```python
from build123d import *

# Parameters (mm, degrees)
SKETCH1_R           = 10.1
BOSS_EXTRUDE1_DEPTH = 13
SKETCH2_R           = 14
BOSS_EXTRUDE2_DEPTH = 3
SKETCH3_R           = 2
CUT_EXTRUDE1_DEPTH  = 17
CIRPATTERN1_COUNT   = 4


with BuildPart() as part:
    # Sketch1 → Boss-Extrude1 (new body)
    with BuildSketch(Plane(origin=(0, 0, 0), x_dir=(1, 0, 0), z_dir=(0, 1, 0))):
        Circle(SKETCH1_R)
    extrude(amount=BOSS_EXTRUDE1_DEPTH)

    # Sketch2 → Boss-Extrude2 (add)
    with BuildSketch(Plane(origin=(0, 13, 0), x_dir=(1, 0, 0), z_dir=(0, 1, 0))):
        Circle(SKETCH2_R)
    extrude(amount=BOSS_EXTRUDE2_DEPTH)

    # Sketch3 → Cut-Extrude1 (cut, through all)
    with BuildSketch(Plane.XZ):
        with Locations((0, 6)):
            Circle(SKETCH3_R)
    cut_extrude1 = extrude(amount=-CUT_EXTRUDE1_DEPTH, mode=Mode.SUBTRACT)

    # CirPattern1: Cut-Extrude1 ×4 about axis
    cirpattern1_axis = Axis((0, 0, 0), (0, 1, 0))
    for i in range(1, CIRPATTERN1_COUNT):
        add(cut_extrude1.rotate(cirpattern1_axis, i * 360 / CIRPATTERN1_COUNT), mode=Mode.SUBTRACT)


solid = part.part
```
CAD build for the part. Positions are in the model's coordinates, mm. A direction names the side the tool comes from. Give positions to 0.01 mm unless a question says otherwise; leave off trailing zeros. Write each loop counter-clockwise with the first axis right and the second up, starting at its lowest first coordinate (ties: lowest second). Pieces come first, ordered by that corner, then holes. Notation, with made-up numbers: M -27,-1 L -10,-1 A25 ccw -10,11 Z; hole C 20.5,28 d7. An arc over 180 degrees is marked long. Return JSON: item names as keys, results as strings. Group by question number.
(1) Band-saw the part on C-C (x = 0). Give the cut face in (y, z).
(2) 3-axis set-ups, long thin cutter, end or side, ignore diameter. For faces 4 (the face through (7.2, 13, -7.3)), 5 (the face through (8, 8, 0)): which of +Z, -Z, +X, -X, +Y, -Y reach the whole face in a straight line?
(3) Drill centre lines: L1, parallel to X at y = 5.25, z = 0; L2, parallel to Y at x = 12.75, z = -2.5. Where is each one in solid material? Low to high. Write a range as [from, to].
(4) Flat gauge pins, fed straight in: pin 1 Ø3 at (x, z) = (-6, 0) entering from -Y; pin 2 Ø1 at (y, z) = (7.5, 1) entering from +X; pin 3 Ø1 at (x, y) = (-7, 9) entering from -Z; pin 4 Ø3 at (x, y) = (0.5, 9) entering from +Z. Where does each tip first touch, or does it go through?
(5) Mould opens along Z. For faces 1 (the face through (9.634, 6.409, -3.034)), 2 (the face through (0, 0, 0)), 3 (the face through (0, 8, -8)) say: pulls with the +Z half, pulls with the -Z half, needs draft (parallel to the pull), parting line crosses it, or undercut.
(6) Band-saw the part on A-A (z = 0). Give the cut face in (x, y).
(7) Band-saw the part on D-D (y = 11.25). Give the cut face in (x, z).
(8) Band-saw the part on B-B (x = -6.5). Give the cut face in (y, z), and give its area (3 significant figures).
Entries:
{
 "1": {"outline": "M 0,-10.1 L 13,-10.1 L 13,-14 L 16,-14 L 16,-8 L 0,-8 Z; M 0,-4 L 16,-4 L 16,4 L 0,4 Z; M 0,8 L 16,8 L 16,14 L 13,14 L 13,10.1 L 0,10.1 Z"},
 "2": {"face 4": "-Y", "face 5": "+Y, -Y"},
 "3": {"L1": "x = [-10.1, -8], [-4, 4], [8, 10.1]", "L2": "y = [13, 16]"},
 "4": {"pin 1": "passes through", "pin 2": "stops at x = 10.09", "pin 3": "stops at z = -7.73", "pin 4": "stops at z = 10.1"},
 "5": {"face 1": "parting line crosses it", "face 2": "needs draft", "face 3": "undercut"},
 "6": {"outline": "M -14,13 L -10.1,13 L -10.1,0 L -8,0 L -8,16 L -14,16 Z; M -4,0 L 4,0 L 4,16 L -4,16 Z; M 8,0 L 10.1,0 L 10.1,13 L 14,13 L 14,16 L 8,16 Z"},
 "7": {"outline": "C 0,0 d20.2; hole C -6,0 d4; hole C 0,-6 d4; hole C 0,6 d4; hole C 6,0 d4"},
 "8": {"outline": "M 0,-7.73 L 13,-7.73 L 13,-12.4 L 16,-12.4 L 16,-1.94 L 0,-1.94 Z; M 0,1.94 L 16,1.94 L 16,12.4 L 13,12.4 L 13,7.73 L 0,7.73 Z", "area": "213 mm^2"}
}
